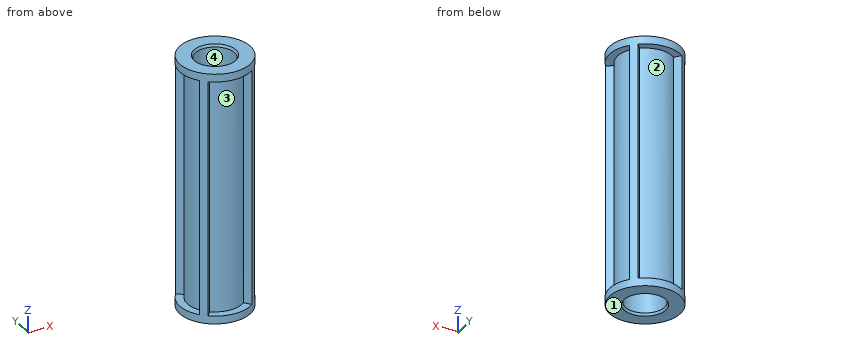
```python
from build123d import *

# Parameters (mm, degrees)
F0_R            = 7.14375
F0_R_2          = 3.96875
F1_DEPTH        = 50.8
F2_SIZE2        = 0.254
F2_SIZE         = 0.508
F6_DEPTH        = 47.625
F6_COPIES_COUNT = 4


# Not quite as in the source:
# - a pattern or mirror of a feature is missing from the dataset's text; its kind, count and spacing are read off the source's solid


with BuildPart() as f1:
    # F0 (on Top) → F1 (new body)
    with BuildSketch(Plane.XY):
        Circle(F0_R)
        Circle(F0_R_2, mode=Mode.SUBTRACT)
    extrude(amount=F1_DEPTH)

    # F2
    f2_edges = [f1.edges().sort_by_distance(p)[0] for p in [
        (-3.96875, 0, 50.8),
        (-3.96875, 0, 0),
    ]]
    f2_side = f1.faces().sort_by_distance((-3.96875, 0, 25.4))[0]
    chamfer(f2_edges, length=F2_SIZE, length2=F2_SIZE2, reference=f2_side)

    # F4 (on offset) → F6 (cut, through all)
    with BuildSketch(Plane(origin=(0, 0, 1.5875), x_dir=(1, 0, 0), z_dir=(0, 0, -1))):
        with BuildLine():
            ThreePointArc((-4.3404758524, -3.4687437838), (-5.55625, 0), (-4.3404758524, 3.4687437838))
            Line((-4.3404758524, 3.4687437838), (-5.5806118102, 4.4598134363))
            ThreePointArc((-5.5806118102, 4.4598134363), (-7.14375, 0), (-5.5806118102, -4.4598134363))
            Line((-5.5806118102, -4.4598134363), (-4.3404758524, -3.4687437838))
        make_face()
    f6 = extrude(amount=-F6_DEPTH, mode=Mode.SUBTRACT)

    # F6_copies: F6 ×4 about axis
    f6_copies_axis = Axis((0, 0, 0), (0, 0, 1))
    for i in range(1, F6_COPIES_COUNT):
        add(f6.rotate(f6_copies_axis, i * 360 / F6_COPIES_COUNT), mode=Mode.SUBTRACT)


solid = f1.part
```
Part model, mm, in its own coordinate system. Face numbers are marked on the shaded views. A direction names the side the tool comes from. Coordinates: 2 decimals unless noted, no trailing zeros. Order: outer loops, then holes, each group sorted by start corner. A loop starts at its lowest first (then second) coordinate and runs counter-clockwise, first axis right, second up. Notation, with made-up numbers: (-27, 59) -> (32, 59) arc R14 ccw to (32, 66) -> close; hole circle Ø7 at (9.25, 25). An arc over 180 degrees is marked (long way). Put each result on its own line as item: value. Start each with the question number.
(1) Pin check, flat tips, straight feed: pin 1 Ø3 at (y, z) = (2, 34) entering from +X; pin 2 Ø5 at (x, z) = (4, 16.5) entering from +Y; pin 3 Ø7 at (x, y) = (0, 0) entering from +Z; pin 4 Ø1 at (y, z) = (-3, 26.5) entering from -X. Stop position of each tip, or through.
(2) Which spindle directions (+Z, -Z, +X, -X, +Y, -Y) get a long thin tool onto all of the face, cutting with end or side? Do the marked faces 3 and 4. Say none if no direction does.
(3) Probe line 1 along X through (y, z) = (0.25, 6); line 2 along Z through (x, y) = (6, 2.75); line 3 along Y through (x, z) = (0, 11). List the from-to ranges inside material, lowest first. Write a range as [from, to].
(4) Mould opens along X. For the marked faces 1 and 2 say: pulls with the +X half, pulls with the -X half, needs draft (parallel to the pull), parting line crosses it, or undercut.
(5) Band-saw the part on B-B (z = 18.5). Give the cut face in (x, y), then the cut area to 3 significant figures.
(6) Band-saw the part on A-A (y = 0). Give the cut face in (x, z), then the cut area to 3 significant figures.
Determined:
1. pin 1: stops at x = 5.53
1. pin 2: stops at y = 5.58
1. pin 3: passes through
1. pin 4: stops at x = -4.96
2. face 3: -Y
2. face 4: +Z, -Z
3. line 1: x = [-5.55, -3.96], [3.96, 5.55]
3. line 2: z = [0, 1.59], [49.21, 50.8]
3. line 3: y = [-5.56, -3.97], [3.97, 5.56]
4. face 1: needs draft
4. face 2: undercut
5. outline: (-5.58, -4.46) arc R7.14 ccw to (-4.46, -5.58) -> (-3.47, -4.34) arc R5.56 ccw to (3.47, -4.34) -> (4.46, -5.58) arc R7.14 ccw to (5.58, -4.46) -> (4.34, -3.47) arc R5.56 ccw to (4.34, 3.47) -> (5.58, 4.46) arc R7.14 ccw to (4.46, 5.58) -> (3.47, 4.34) arc R5.56 ccw to (-3.47, 4.34) -> (-4.46, 5.58) arc R7.14 ccw to (-5.58, 4.46) -> (-4.34, 3.47) arc R5.56 ccw to (-4.34, -3.47) -> close; hole circle Ø7.94 at (0, 0)
5. area: 56.5 mm²
6. outline: (-7.14, 0) -> (-4.22, 0) -> (-3.97, 0.51) -> (-3.97, 50.29) -> (-4.22, 50.8) -> (-7.14, 50.8) -> (-7.14, 49.21) -> (-5.56, 49.21) -> (-5.56, 1.59) -> (-7.14, 1.59) -> close; (3.97, 0.51) -> (4.22, 0) -> (7.14, 0) -> (7.14, 1.59) -> (5.56, 1.59) -> (5.56, 49.21) -> (7.14, 49.21) -> (7.14, 50.8) -> (4.22, 50.8) -> (3.97, 50.29) -> close
6. area: 171 mm²
